The drawing under review shows one solid part. Ordinate dimensions are in mm from its lowest x, y, z. A direction names the side the tool comes from. Round coordinates to 2 decimals unless told otherwise and drop trailing zeros. Write each loop counter-clockwise with the first axis right and the second up, starting at its lowest first coordinate (ties: lowest second). Pieces come first, ordered by that corner, then holes.
Item 1: Clearance check with flat-ended pins moving along their axes: pin 1 Ø1.5 at (x, z) = (20, 5.5) entering from -Y; pin 2 Ø2 at (x, z) = (39.5, 6.5) entering from +Y; pin 3 Ø6 at (x, y) = (7.5, 34.5) entering from +Z; pin 4 Ø1 at (x, z) = (12, 25) entering from +Y. State where each tip first meets the part, or that it passes through.
Item 2: To check wall thickness, follow L1, parallel to X at y = 4, z = 19; L2, parallel to Y at x = 24, z = 20. State the ranges of each line that lie inside material, in increasing order.
Item 3: Add section C-C (x = 9.5). Give the boundary of the cut face in (y, z), plus the area to 3 significant figures.
Item 4: Add section D-D (y = 122). Give the boundary of the cut face in (x, z), plus the area to 3 significant figures.
Item 5: Add section A-A (z = 19.05). Give the boundary of the cut face in (x, y) (3 decimals).
Item 6: Add section B-B (z = 5). Give the boundary of the cut face in (x, y) (3 decimals), plus the area to 3 significant figures.
Item 7: Machinability: for the marked faces 1 and 2, which of the approach directions +Z, -Z, +X, -X, +Y, -Y give a long, thin tool a straight path to every point of the face, cutting with its end or side? Answer none if there is none.
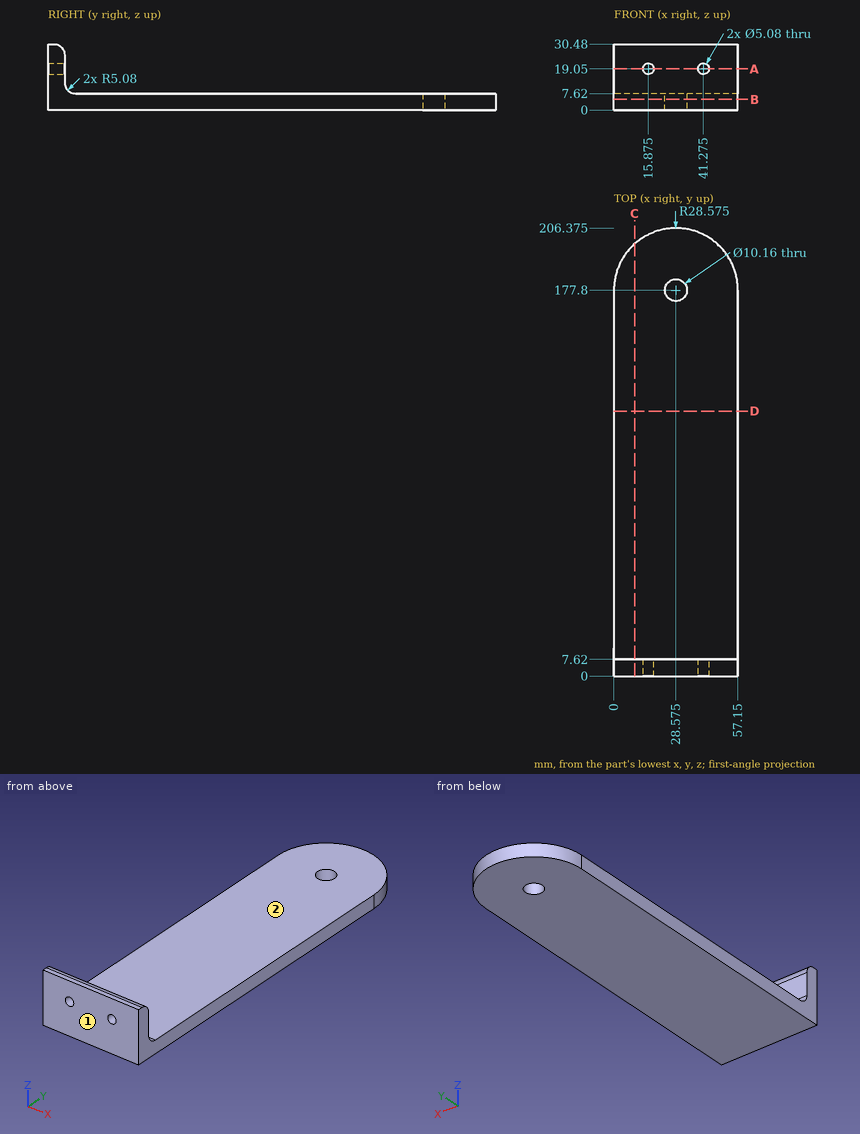
Numbers:
1. pin 1: stops at y = 0
1. pin 2: stops at y = 204.6
1. pin 3: stops at z = 7.62
1. pin 4: stops at y = 7.62
2. L1: x = 0 to 13.34, 18.41 to 38.74, 43.81 to 57.15
2. L2: y = 0 to 7.62
3. outline: (0, 0) - (199.08, 0) - (199.08, 7.62) - (12.7, 7.62) arc R5.08 cw to (7.62, 12.7) - (7.62, 25.4) arc R5.08 ccw to (2.54, 30.48) - (0, 30.48) - close
3. area: 1,690 mm2
4. outline: (0, 0) - (57.15, 0) - (57.15, 7.62) - (0, 7.62) - close
4. area: 435 mm2
5. outline: (0, 0) - (13.335, 0) - (13.335, 7.62) - (0, 7.62) - close; (18.415, 0) - (38.735, 0) - (38.735, 7.62) - (18.415, 7.62) - close; (43.815, 0) - (57.15, 0) - (57.15, 7.62) - (43.815, 7.62) - close
6. outline: (0, 0) - (57.15, 0) - (57.15, 177.8) arc R28.575 ccw to (0, 177.8) - close; hole circle Ø10.16 at (28.575, 177.8)
6. area: 11,400 mm2
7. face 1: +Z, -Z, +X, -X, -Y
7. face 2: +Z, +X, -X, +Y
